```python
from build123d import *

# Parameters (mm, degrees)
F1_R     = 10
F1_R_2   = 7
F2_DEPTH = 2
F1_R_3   = 6.05
F3_DEPTH = 10
F4_SIZE  = 0.8


with BuildPart() as f2:
    # F1 (on Top) → F2 (new body)
    with BuildSketch(Plane.XY):
        Circle(F1_R)
        Circle(F1_R_2, mode=Mode.SUBTRACT)
    extrude(amount=F2_DEPTH)

    # F1 (on Top) → F3 (join)
    with BuildSketch(Plane.XY):
        Circle(F1_R_2)
        Circle(F1_R_3, mode=Mode.SUBTRACT)
    extrude(amount=F3_DEPTH)

    # F4
    f4_edges = [f2.edges().sort_by_distance(p)[0] for p in [
        (-6.05, 0, 0),
    ]]
    chamfer(f4_edges, length=F4_SIZE)


solid = f2.part
```
Work out the finished part from the listing and answer in its coordinate system (mm). Give positions to 0.01 mm unless a question says otherwise; leave off trailing zeros. Loops run counter-clockwise (first coordinate to the right, second up) from the corner with the lowest first, then second, coordinate; pieces in that order, holes last. Notation, with made-up numbers: (38.5, 62) -> (68.5, 62) arc R18 ccw to (68.5, 76) -> close; hole circle Ø5 at (-9, 75). An arc over 180 degrees is marked (long way). Put each result on its own line as item: value. Start each with the question number.
Item 1: The mould has two halves that part along Y. Classify faces 1 (the face through (5.589, -2.317, 5.336)), 2 (the face through (-7, -2, 2)), 3 (the face through (6.466, -2.681, 5.944)): released by +Y, released by -Y, zero draft, split by the parting line, or undercut.
Item 2: Each of these flat-tipped pins is pushed along its axis until it touches: P1, Ø1.5, axis at x = -5.5, z = 2.5, coming from the -Y side; P2, Ø6, axis at y = -4, z = 7.5, coming from the -X side; P3, Ø6, axis at y = 5, z = 2.5, coming from the -X side. Where does it stop, or does it pass through?
Item 3: The part is cut by section B-B (z = 2.25). Give the vertices of the cut face in (x, y), then the cut area to 3 significant figures.
Item 4: The part is cut by section A-A (x = 0). Give the vertices of the cut face in (y, z), then the cut area to 3 significant figures.
Item 5: The part is cut by section C-C (y = 7.5). Give the vertices of the cut face in (x, z), then the cut area to 3 significant figures.
Item 6: Find the intervals of material crossed by L1, parallel to Y at x = 0, z = 3; L2, parallel to Z at x = 5.25, y = -6.25; L3, parallel to Y at x = 4.75, z = 6, in increasing order. Write a range as [from, to].
Answers below:
1. face 1: undercut
1. face 2: zero draft
1. face 3: split by the parting line
2. P1: y = -8.69
2. P2: x = -6.93
2. P3: x = -9.79
3. outline: circle Ø14 at (0, 0); hole circle Ø12.1 at (0, 0)
3. area: 38.9 mm2
4. outline: (-10, 0) -> (-6.85, 0) -> (-6.05, 0.8) -> (-6.05, 10) -> (-7, 10) -> (-7, 2) -> (-10, 2) -> close; (6.05, 0.8) -> (6.85, 0) -> (10, 0) -> (10, 2) -> (7, 2) -> (7, 10) -> (6.05, 10) -> close
4. area: 30.4 mm2
5. outline: (-6.61, 0) -> (6.61, 0) -> (6.61, 2) -> (-6.61, 2) -> close
5. area: 26.5 mm2
6. L1: [-7, -6.05], [6.05, 7]
6. L2: [0, 2]
6. L3: [-5.14, -3.75], [3.75, 5.14]
